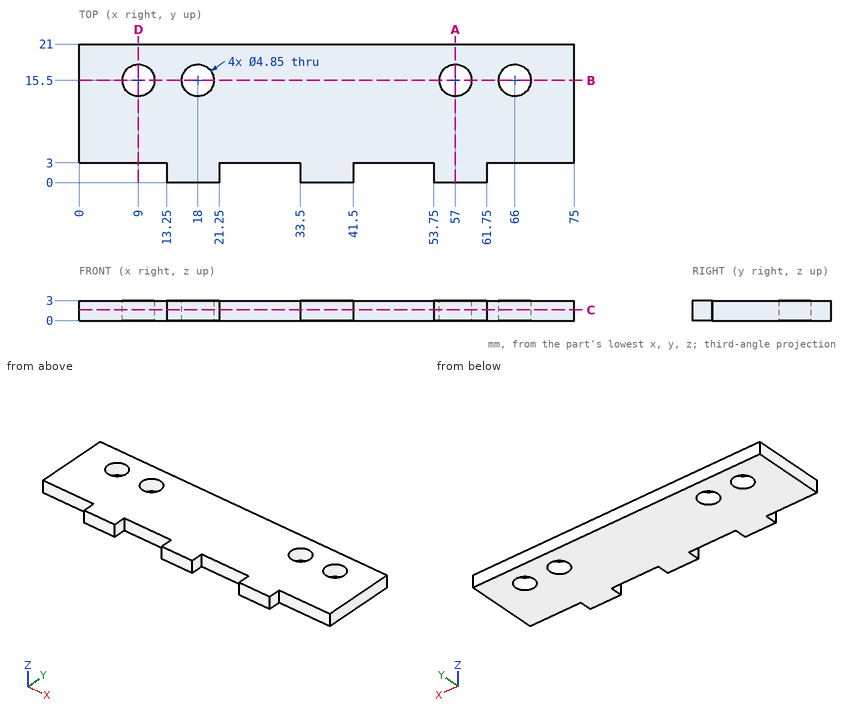
Part print with two shaded views. Sizes in mm from the minimum x, y, z corner. Round coordinates to 2 decimals unless told otherwise and drop trailing zeros. Loops run counter-clockwise (first coordinate to the right, second up) from the corner with the lowest first, then second, coordinate; pieces in that order, holes last.
1. Slice it at B-B (y = 15.5). Give the cut face in (x, z) (3 decimals), and give its area (3 significant figures).
Solutions:
outline: (0, 0) - (6.575, 0) - (6.575, 3) - (0, 3) - close; (11.425, 0) - (15.575, 0) - (15.575, 3) - (11.425, 3) - close; (20.425, 0) - (54.575, 0) - (54.575, 3) - (20.425, 3) - close; (59.425, 0) - (63.575, 0) - (63.575, 3) - (59.425, 3) - close; (68.425, 0) - (75, 0) - (75, 3) - (68.425, 3) - close
area: 167 mm2
2. Slice it at D-D (x = 9). Give the cut face in (y, z) (3 decimals), and give its area (4 significant figures).
Solutions:
outline: (3, 0) - (13.075, 0) - (13.075, 3) - (3, 3) - close; (17.925, 0) - (21, 0) - (21, 3) - (17.925, 3) - close
area: 39.45 mm2
3. Slice it at A-A (x = 57). Give the cut face in (y, z) (3 decimals), and give its area (4 significant figures).
Solutions:
outline: (0, 0) - (13.075, 0) - (13.075, 3) - (0, 3) - close; (17.925, 0) - (21, 0) - (21, 3) - (17.925, 3) - close
area: 48.45 mm2
4. Flat gauge pins, fed straight in: pin 1 (3 mm diameter, centred on x = 18, y = 15.5, fed in from +Z) (3 decimals); pin 2 (1.5 mm diameter, centred on x = 4, z = 1, fed in from -Y); pin 3 (1 mm diameter, centred on x = 38.5, z = 2.5, fed in from -Y); pin 4 (0.9 mm diameter, centred on y = 1, z = 2, fed in from +X). Where does each tip first touch, or does it go through?
Solutions:
pin 1: passes through
pin 2: stops at y = 3
pin 3: stops at y = 0
pin 4: stops at x = 61.75
5. Drill centre lines: line 1 along Y through (x, z) = (57, 2) (3 decimals); line 2 along X through (y, z) = (2.75, 1.2); line 3 along Y through (x, z) = (9, 1.4) (3 decimals). Where is each one in solid material? Low to high.
Solutions:
line 1: y = 0 to 13.075, 17.925 to 21
line 2: x = 13.25 to 21.25, 33.5 to 41.5, 53.75 to 61.75
line 3: y = 3 to 13.075, 17.925 to 21
6. Slice it at C-C (z = 1.6). Give the cut face in (x, y) (3 decimals).
Solutions:
outline: (0, 3) - (13.25, 3) - (13.25, 0) - (21.25, 0) - (21.25, 3) - (33.5, 3) - (33.5, 0) - (41.5, 0) - (41.5, 3) - (53.75, 3) - (53.75, 0) - (61.75, 0) - (61.75, 3) - (75, 3) - (75, 21) - (0, 21) - close; hole circle Ø4.85 at (9, 15.5); hole circle Ø4.85 at (18, 15.5); hole circle Ø4.85 at (57, 15.5); hole circle Ø4.85 at (66, 15.5)
